Read the model definition and answer for the solid it produces. Units are mm, in the model's axes. A direction names the side the tool comes from. Coordinates: 2 decimals unless noted, no trailing zeros. Write each loop counter-clockwise with the first axis right and the second up, starting at its lowest first coordinate (ties: lowest second). Pieces come first, ordered by that corner, then holes.
1) The part is cut by section B-B (x = 0). Determine the outline of the cut face in (y, z).
2) Determine the mould class of faces 1 (the face through (2.192, -23.269, -4.214)), 2 (the face through (3.233, -3.451, -1.341)), 3 (the face through (-0.75, -20.48, 5.7)), 4 (the face through (2.6, -1.5, -5.4)) for opening direction X: +X half, -X half, draft (parallel to the pull), parting line (faces both ways), or undercut.
3) Find the intervals of material crossed by line 1 (Z direction, x = 0, y = -32.5); line 2 (Z direction, x = 0, y = -4.75); line 3 (Y direction, x = -6.5, z = 4.25), in increasing order.
4) The part is cut by section D-D (x = 9.5). Determine the outline of the cut face in (y, z), then the cut area to 3 significant figures.
5) Each of these flat-tipped pins is pushed along its axis until it touches: pin 1 Ø1.5 at (y, z) = (-10.5, 5) entering from -X; pin 2 Ø2 at (x, y) = (-3.5, -11) entering from -Z; pin 3 Ø10 at (y, z) = (-17, 4.5) entering from +X; pin 4 Ø1.5 at (y, z) = (-22, 7.5) entering from +X. Where does it stop, or does it pass through?
6) The part is cut by section C-C (y = -33). Determine the outline of the cut face in (x, z), then the cut area to 3 significant figures.
7) The part is cut by section A-A (z = 0). Determine the outline of the cut face in (x, y), then the cut area to 3 significant figures.
8) Which of the six approach directions +Z, -Z, +X, -X, +Y, -Y give full straight-line access (tool end or side, diameter ignored) to faces 5 (the face through (11.923, -0.74, 3.755)), 6 (the face through (-4, -7, 0))?
from build123d import *

# Parameters (mm, degrees)
F0_R     = 5.75
F0_R_2   = 4.75
F0_R_3   = 12.5
F1_DEPTH = 1.5
F2_DEPTH = 40
F0_R_4   = 3.5
F3_DEPTH = 7


with BuildPart() as f1:
    # F0 (on Front) → F1 (new body)
    with BuildSketch(Plane.XZ):
        Circle(F0_R)
        Circle(F0_R_2, mode=Mode.SUBTRACT)
        Circle(F0_R_3)
        Circle(F0_R, mode=Mode.SUBTRACT)
    extrude(amount=F1_DEPTH)

    # F0 (on Front) → F2 (join)
    with BuildSketch(Plane.XZ):
        Circle(F0_R)
        Circle(F0_R_2, mode=Mode.SUBTRACT)
    extrude(amount=F2_DEPTH)

    # F0 (on Front) → F3 (join)
    with BuildSketch(Plane.XZ):
        Circle(F0_R_2)
        Circle(F0_R_4, mode=Mode.SUBTRACT)
    extrude(amount=F3_DEPTH)


solid = f1.part
Reported:
1. outline: (-40, -5.75) - (-1.5, -5.75) - (-1.5, -12.5) - (0, -12.5) - (0, -3.5) - (-7, -3.5) - (-7, -4.75) - (-40, -4.75) - close; (-40, 4.75) - (-7, 4.75) - (-7, 3.5) - (0, 3.5) - (0, 12.5) - (-1.5, 12.5) - (-1.5, 5.75) - (-40, 5.75) - close
2. face 1: undercut
2. face 2: undercut
2. face 3: parting line
2. face 4: draft
3. line 1: z = -5.75 to -4.75, 4.75 to 5.75
3. line 2: z = -5.75 to -3.5, 3.5 to 5.75
3. line 3: y = -1.5 to 0
4. outline: (-1.5, -8.12) - (0, -8.12) - (0, 8.12) - (-1.5, 8.12) - close
4. area: 24.4 mm2
5. pin 1: stops at x = -3.87
5. pin 2: stops at z = -5.18
5. pin 3: stops at x = 5.75
5. pin 4: passes through
6. outline: circle Ø11.5 at (0, 0); hole circle Ø9.5 at (0, 0)
6. area: 33.0 mm2
7. outline: (-12.5, -1.5) - (-5.75, -1.5) - (-5.75, -40) - (-4.75, -40) - (-4.75, -7) - (-3.5, -7) - (-3.5, 0) - (-12.5, 0) - close; (3.5, -7) - (4.75, -7) - (4.75, -40) - (5.75, -40) - (5.75, -1.5) - (12.5, -1.5) - (12.5, 0) - (3.5, 0) - close
7. area: 118 mm2
8. face 5: +Y, -Y
8. face 6: -Y
